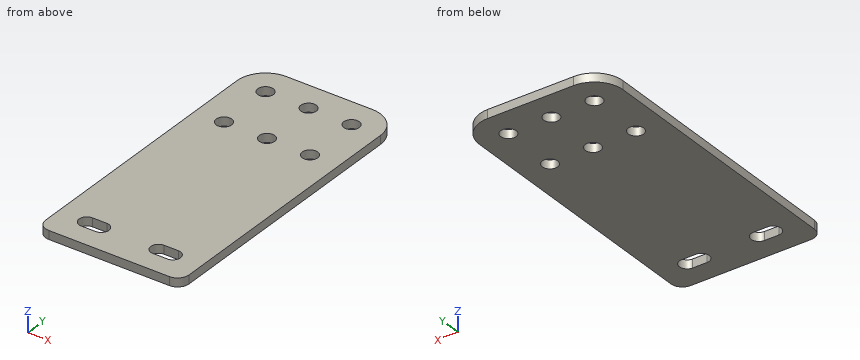
from build123d import *

# Parameters (mm, degrees)
MODEL_R                         = 2.7
AUFSATZ_LINEAR_AUSTRAGEN1_DEPTH = 3


with BuildPart() as part:
    # Model → Aufsatz-Linear austragen1 (new body)
    with BuildSketch(Plane.XY):
        with BuildLine():
            Line((40, 106), (10, 106))
            ThreePointArc((10, 106), (2.928932188, 103.071067812), (0, 96))
            Line((0, 96), (0, 4))
            ThreePointArc((0, 4), (1.171572875, 1.171572875), (4, 0))
            Line((4, 0), (46, 0))
            ThreePointArc((46, 0), (48.828427125, 1.171572875), (50, 4))
            Line((50, 4), (50, 96))
            ThreePointArc((50, 96), (47.071067812, 103.071067812), (40, 106))
        make_face()
        with Locations((25, 76)):
            Circle(MODEL_R, mode=Mode.SUBTRACT)
        with Locations((25, 96)):
            Circle(MODEL_R, mode=Mode.SUBTRACT)
        with Locations((40, 76)):
            Circle(MODEL_R, mode=Mode.SUBTRACT)
        with Locations((40, 96)):
            Circle(MODEL_R, mode=Mode.SUBTRACT)
        with Locations((10, 76)):
            Circle(MODEL_R, mode=Mode.SUBTRACT)
        with Locations((10, 96)):
            Circle(MODEL_R, mode=Mode.SUBTRACT)
        with BuildLine():
            Line((15, 7.3), (10, 7.3))
            ThreePointArc((10, 7.3), (7.3, 10), (10, 12.7))
            Line((10, 12.7), (15, 12.7))
            ThreePointArc((15, 12.7), (17.7, 10), (15, 7.3))
        make_face(mode=Mode.SUBTRACT)
        with BuildLine():
            Line((40, 7.3), (35, 7.3))
            ThreePointArc((35, 7.3), (32.3, 10), (35, 12.7))
            Line((35, 12.7), (40, 12.7))
            ThreePointArc((40, 12.7), (42.7, 10), (40, 7.3))
        make_face(mode=Mode.SUBTRACT)
    extrude(amount=AUFSATZ_LINEAR_AUSTRAGEN1_DEPTH)


solid = part.part
Design review of the part built by this model. Coordinates are the model's own, in mm. Round coordinates to 2 decimals unless told otherwise and drop trailing zeros. Write each loop counter-clockwise with the first axis right and the second up, starting at its lowest first coordinate (ties: lowest second). Pieces come first, ordered by that corner, then holes. Notation, with made-up numbers: (0.5, 20.5) - (46.5, 20.5) arc R24 cw to (46.5, 49.5) - close; hole circle Ø8 at (-33.5, 77). An arc over 180 degrees is marked (long way). Use a Markdown table: item, result. Add a question column.
1. Wall thickness on probe 1 along Y at (x, z) = (40, 1.25); probe 2 along Y at (x, z) = (25, 2.35); probe 3 along Y at (x, z) = (41, 0.2): over which ranges is each line inside the solid? List them lowest first.
2. We need section C-C (x = 25). State the section outline as (y, z) points, then the cut area to 3 significant figures.
3. We need section A-A (y = 10). State the section outline as (x, z) points, then the cut area to 3 significant figures.
4. We need section B-B (z = 1.55). Count the separate pieces of the cut face and the enclosed holes in it, then the cut area to 3 significant figures.
5. Clearance check with a flat-ended pin moving along its axis: pin 1 (4.5 mm diameter, centred on x = 10, y = 76, fed in from -Z). State where the tip first meets the part, or that it passes through.
6. We need section D-D (x = 39). State the section outline as (y, z) points, then the cut area to 3 significant figures.
Output:
| question | item | result |
|---|---|---|
| 1 | probe 1 | y = 0 to 7.3, 12.7 to 73.3, 78.7 to 93.3, 98.7 to 106 |
| 1 | probe 2 | y = 0 to 73.3, 78.7 to 93.3, 98.7 to 106 |
| 1 | probe 3 | y = 0 to 7.49, 12.51 to 73.49, 78.51 to 93.49, 98.51 to 105.95 |
| 2 | outline | (0, 0) - (73.3, 0) - (73.3, 3) - (0, 3) - close; (78.7, 0) - (93.3, 0) - (93.3, 3) - (78.7, 3) - close; (98.7, 0) - (106, 0) - (106, 3) - (98.7, 3) - close |
| 2 | area | 286 mm2 |
| 3 | outline | (0, 0) - (7.3, 0) - (7.3, 3) - (0, 3) - close; (17.7, 0) - (32.3, 0) - (32.3, 3) - (17.7, 3) - close; (42.7, 0) - (50, 0) - (50, 3) - (42.7, 3) - close |
| 3 | area | 87.6 mm2 |
| 4 | separate pieces | 1 |
| 4 | enclosed holes | 8 |
| 4 | area | 5,010 mm2 |
| 5 | pin 1 | passes through |
| 6 | outline | (0, 0) - (7.3, 0) - (7.3, 3) - (0, 3) - close; (12.7, 0) - (73.49, 0) - (73.49, 3) - (12.7, 3) - close; (78.51, 0) - (93.49, 0) - (93.49, 3) - (78.51, 3) - close; (98.51, 0) - (106, 0) - (106, 3) - (98.51, 3) - close |
| 6 | area | 272 mm2 |
